Build history of the part. All positions in model axes, mm. Face numbers are marked on the shaded views. A direction names the side the tool comes from. Round coordinates to 2 decimals unless told otherwise and drop trailing zeros. Write each loop counter-clockwise with the first axis right and the second up, starting at its lowest first coordinate (ties: lowest second). Pieces come first, ordered by that corner, then holes. Notation, with made-up numbers: M -14.75,57 L 38.25,57 A33 cw 38.25,89 Z; hole C 27.25,-34.75 d3. An arc over 180 degrees is marked long. Use a Markdown table: item, result.
from build123d import *

# Parameters (mm, degrees)
SKETCH_1_W          = 10
SKETCH_1_H          = 15.4
EXTRUDE_1_DEPTH     = 4.5
SKETCH_2_W          = 10
SKETCH_2_H          = 6.5
CUT_EXTRUDE_1_DEPTH = 3.3
CHAMFER_1_SIZE      = 2
SKETCH_3_R          = 1.75
CUT_EXTRUDE_2_DEPTH = 17.524224641
SKETCH_4_W          = 0.965597518
SKETCH_4_H          = 0.5
EXTRUDE_2_DEPTH     = 13


with BuildPart() as part:
    # 草图1 → 凸台-拉伸1 (new body)
    with BuildSketch(Plane.XY):
        with Locations((0, 7.7)):
            Rectangle(SKETCH_1_W, SKETCH_1_H)
    extrude(amount=EXTRUDE_1_DEPTH)

    # 草图2 → 切除-拉伸1 (cut)
    with BuildSketch(Plane.XY.offset(4.5)):
        with Locations((0, 12.15)):
            Rectangle(SKETCH_2_W, SKETCH_2_H)
    extrude(amount=-CUT_EXTRUDE_1_DEPTH, mode=Mode.SUBTRACT)

    # 倒角1
    chamfer_1_edges = [part.edges().sort_by_distance(p)[0] for p in [
        (0, 8.9, 4.5),
    ]]
    chamfer(chamfer_1_edges, length=CHAMFER_1_SIZE)

    # 草图3 → 切除-拉伸2 (cut, through all)
    with BuildSketch(Plane.XY.offset(1.2)):
        with Locations((0, 12.4)):
            Circle(SKETCH_3_R)
    extrude(amount=-CUT_EXTRUDE_2_DEPTH, mode=Mode.SUBTRACT)

    # 草图4 → 凸台-拉伸2 (add)
    with BuildSketch(Plane.XZ):
        with Locations((2.54, 3.23)):
            Rectangle(SKETCH_4_W, SKETCH_4_H)
        with Locations((0, 3.23)):
            Rectangle(SKETCH_4_W, SKETCH_4_H)
        with Locations((-2.54, 3.23)):
            Rectangle(SKETCH_4_W, SKETCH_4_H)
    extrude(amount=EXTRUDE_2_DEPTH)


solid = part.part
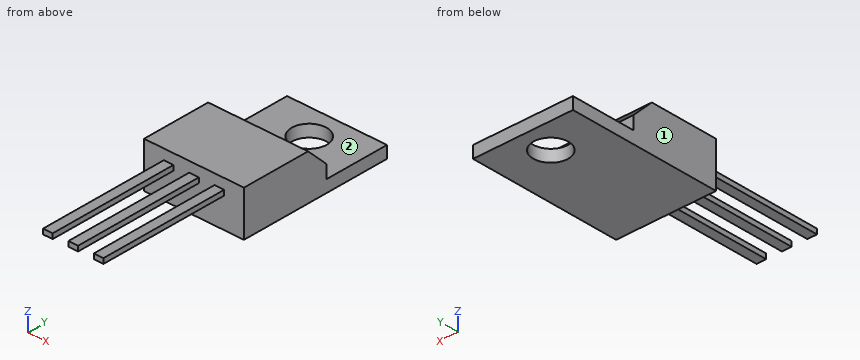
Q1. Cut at C-C on y = -1.25. Give the cut face in (x, z), and give its area (3 significant figures).
Response values:
| item | result |
|---|---|
| outline | M -3.02,2.98 L -2.06,2.98 L -2.06,3.48 L -3.02,3.48 Z; M -0.48,2.98 L 0.48,2.98 L 0.48,3.48 L -0.48,3.48 Z; M 2.06,2.98 L 3.02,2.98 L 3.02,3.48 L 2.06,3.48 Z |
| area | 1.45 mm2 |
Q2. Drop flat-ended pins along their axis: P1, Ø2, axis at x = 3.5, y = 9.5, coming from the -Z side; P2, Ø0.8, axis at x = 0, y = -4, coming from the -Z side; P3, Ø0.5, axis at x = -2.5, y = -5.5, coming from the +Z side; P4, Ø0.6, axis at y = -8.5, z = 3, coming from the +X side. Give the stop position or say it passes through.
Response values:
| item | result |
|---|---|
| P1 | stops at z = 0 |
| P2 | stops at z = 2.98 |
| P3 | stops at z = 3.48 |
| P4 | stops at x = 3.02 |
Q3. Cut at A-A on y = 12.4. Give the cut face in (x, z).
Response values:
| item | result |
|---|---|
| outline | M -5,0 L -1.75,0 L -1.75,1.2 L -5,1.2 Z; M 1.75,0 L 5,0 L 5,1.2 L 1.75,1.2 Z |
Q4. Cut at B-B on x = 0. Give the cut face in (y, z), and give its area (4 significant figures).
Response values:
| item | result |
|---|---|
| outline | M -13,2.98 L 0,2.98 L 0,0 L 10.65,0 L 10.65,1.2 L 8.9,1.2 L 8.9,2.5 L 6.9,4.5 L 0,4.5 L 0,3.48 L -13,3.48 Z; M 14.15,0 L 15.4,0 L 15.4,1.2 L 14.15,1.2 Z |
| area | 48.15 mm2 |
Q5. Drill centre lines: L1, parallel to Y at x = 0, z = 0.45; L2, parallel to Z at x = -1.25, y = 10.5; L3, parallel to Y at x = 1.5, z = 2.1. Where is each one in solid material? Low to high.
Response values:
| item | result |
|---|---|
| L1 | y = 0 to 10.65, 14.15 to 15.4 |
| L2 | z = 0 to 1.2 |
| L3 | y = 0 to 8.9 |
Q6. Which spindle directions (+Z, -Z, +X, -X, +Y, -Y) get a long thin tool onto all of the face, cutting with end or side? Do the marked faces 1 and 2. Say none if no direction does.
Response values:
| item | result |
|---|---|
| face 1 | +Z, -Z, -X, +Y, -Y |
| face 2 | +Z, +X, -X, +Y |
Q7. Cut at D-D on z = 2.2. Give the cut face in (x, y), and give its area (3 significant figures).
Response values:
| item | result |
|---|---|
| outline | M -5,0 L 5,0 L 5,8.9 L -5,8.9 Z |
| area | 89.0 mm2 |
